The model under review builds one solid part; all positions refer to its coordinate system, in mm. Round coordinates to 2 decimals unless told otherwise and drop trailing zeros. Order: outer loops, then holes, each group sorted by start corner. A loop starts at its lowest first (then second) coordinate and runs counter-clockwise, first axis right, second up. Notation, with made-up numbers: M 64,-12.5 L 123,-12.5 A19 ccw 123,5.5 Z; hole C 39.5,-31.5 d8. An arc over 180 degrees is marked long. Use a Markdown table: item, result. Add a question column.
1. To check wall thickness, follow probe 1 along X at (y, z) = (0.25, 263); probe 2 along X at (y, z) = (-4.5, 23.5); probe 3 along Y at (x, z) = (4.5, 245). State the ranges of each line that lie inside material, in increasing order.
2. Consider section A-A on z = 235.5. State the section outline as (x, y) points, then the cut area to 3 significant figures.
3. Insertion check: P1, Ø5, axis at y = -4.5, z = 66.5, coming from the -X side; P2, Ø3, axis at y = 4, z = 223, coming from the +X side; P3, Ø2, axis at y = -4, z = 119, coming from the -X side. Each pin has a flat end and moves straight along its axis. Give the tip position at first contact, or say it passes through.
from build123d import *

# Parameters (mm, degrees)
BOSS_EXTRUDE1_DEPTH = 304.8


with BuildPart() as part:
    # Sketch1 → Boss-Extrude1 (new body)
    with BuildSketch(Plane.XY):
        with BuildLine():
            ThreePointArc((-6.643813628, 1.19257724), (-6.75, 0), (-6.643813628, -1.19257724))
            Line((-6.643813628, -1.19257724), (-4.354709, -5.15742276))
            ThreePointArc((-4.354709, -5.15742276), (-3.375, -5.845671476), (-2.289104628, -6.35))
            Line((-2.289104628, -6.35), (2.289104628, -6.35))
            ThreePointArc((2.289104628, -6.35), (3.375, -5.845671476), (4.354709, -5.15742276))
            Line((4.354709, -5.15742276), (6.643813628, -1.19257724))
            ThreePointArc((6.643813628, -1.19257724), (6.723400999, -0.598647646), (6.75, 0))
            ThreePointArc((6.75, 0), (6.723400999, 0.598647646), (6.643813628, 1.19257724))
            Line((6.643813628, 1.19257724), (4.354709, 5.15742276))
            ThreePointArc((4.354709, 5.15742276), (3.375, 5.845671476), (2.289104628, 6.35))
            Line((2.289104628, 6.35), (-2.289104628, 6.35))
            ThreePointArc((-2.289104628, 6.35), (-3.375, 5.845671476), (-4.354709, 5.15742276))
            Line((-4.354709, 5.15742276), (-6.643813628, 1.19257724))
        make_face()
    extrude(amount=BOSS_EXTRUDE1_DEPTH)


solid = part.part
Answer block:
| question | item | result |
|---|---|---|
| 1 | probe 1 | -6.75 to 6.75 |
| 1 | probe 2 | -4.73 to 4.73 |
| 1 | probe 3 | -4.91 to 4.91 |
| 2 | outline | M -6.64,-1.19 L -4.35,-5.16 A6.75 ccw -2.29,-6.35 L 2.29,-6.35 A6.75 ccw 4.35,-5.16 L 6.64,-1.19 A6.75 ccw 6.64,1.19 L 4.35,5.16 A6.75 ccw 2.29,6.35 L -2.29,6.35 A6.75 ccw -4.35,5.16 L -6.64,1.19 A6.75 ccw Z |
| 2 | area | 136 mm^2 |
| 3 | P1 | x = -6.18 |
| 3 | P2 | x = 5.89 |
| 3 | P3 | x = -5.6 |
